Design review of the part built by this model. Coordinates are the model's own, in mm. A direction names the side the tool comes from. Coordinates: 2 decimals unless noted, no trailing zeros. Loops run counter-clockwise (first coordinate to the right, second up) from the corner with the lowest first, then second, coordinate; pieces in that order, holes last. Notation, with made-up numbers: (13.25, 79.5) -> (35.25, 79.5) arc R13 cw to (35.25, 89.5) -> close; hole circle Ø7 at (71.5, 0). An arc over 180 degrees is marked (long way). Use CSV: the item, a comma, the result in double quotes.
```python
from build123d import *

# Parameters (mm, degrees)
SKETCH1_W               = 95.25
SKETCH1_H               = 65.405
BOSS_EXTRUDE1_DEPTH     = 21.59
SKETCH2_W               = 90.17
SKETCH2_H               = 60.325
CUT_EXTRUDE1_DEPTH      = 21.59
CUT_EXTRUDE2_REACH      = 104.996
SKETCH3_W               = 7
SKETCH3_H               = 3
CUT_EXTRUDE3_DEPTH      = 84.738179763
CUT_EXTRUDE3_DEPTH_BACK = 84.738179763
SKETCH4_W               = 20.32
SKETCH4_H               = 3.81


with BuildPart() as part:
    # Sketch1 → Boss-Extrude1 (new body)
    with BuildSketch(Plane(origin=(0, 0, 0), x_dir=(1, 0, 0), z_dir=(0, 1, 0))):
        Rectangle(SKETCH1_W, SKETCH1_H)
    extrude(amount=BOSS_EXTRUDE1_DEPTH)

    # Sketch2 → Cut-Extrude1 (cut)
    with BuildSketch(Plane(origin=(0, 21.59, 0), x_dir=(1, 0, 0), z_dir=(0, 1, 0))):
        Rectangle(SKETCH2_W, SKETCH2_H)
    extrude(amount=-CUT_EXTRUDE1_DEPTH, mode=Mode.SUBTRACT)

    # Sketch3 → Cut-Extrude2 (cut, up to next)
    with BuildSketch(Plane.ZY.offset(47.625), mode=Mode.PRIVATE) as cut_extrude2_sk1:
        with Locations((0, 5.08)):
            Rectangle(SKETCH3_W, SKETCH3_H)
    cut_extrude2_tool1 = extrude(cut_extrude2_sk1.sketch, amount=-CUT_EXTRUDE2_REACH, mode=Mode.PRIVATE) & part.part
    add(cut_extrude2_tool1.solids().sort_by_distance((-47.625, 5.08, 0))[0], mode=Mode.SUBTRACT)

    # Sketch4 → Cut-Extrude3 (cut, two sides: drawn at the far end of the back side and taken through both)
    with BuildSketch(Plane(origin=(0, 0, -32.7025), x_dir=(-1, 0, 0), z_dir=(0, 0, -1)).offset(-CUT_EXTRUDE3_DEPTH_BACK)):
        with Locations((-31.115, 1.905)):
            Rectangle(SKETCH4_W, SKETCH4_H)
        with Locations((31.115, 1.905)):
            Rectangle(SKETCH4_W, SKETCH4_H)
    extrude(amount=CUT_EXTRUDE3_DEPTH + CUT_EXTRUDE3_DEPTH_BACK, mode=Mode.SUBTRACT)


solid = part.part
```
Item 1: Add section A-A (z = 5.5). Give the boundary of the cut face in (x, y) (3 decimals), then the cut area to 3 significant figures.
Checked values:
outline,"(-47.625, 0) -> (-45.085, 0) -> (-45.085, 21.59) -> (-47.625, 21.59) -> close; (45.085, 0) -> (47.625, 0) -> (47.625, 21.59) -> (45.085, 21.59) -> close"
area,"110 mm^2"
Item 2: Add section B-B (x = -25.5). Give the boundary of the cut face in (y, z).
Checked values:
outline,"(3.81, -32.7) -> (21.59, -32.7) -> (21.59, -30.16) -> (3.81, -30.16) -> close; (3.81, 30.16) -> (21.59, 30.16) -> (21.59, 32.7) -> (3.81, 32.7) -> close"
Item 3: Add section C-C (y = 12). Give the boundary of the cut face in (x, z) (1 decimal), then the cut area to 3 significant figures.
Checked values:
outline,"(-47.6, -32.7) -> (47.6, -32.7) -> (47.6, 32.7) -> (-47.6, 32.7) -> close; hole (-45.1, -30.2) -> (45.1, -30.2) -> (45.1, 30.2) -> (-45.1, 30.2) -> close"
area,"790 mm^2"
Item 4: Clearance check with a flat-ended pin moving along its axis: pin 1 (1.3 mm diameter, centred on x = -31, z = 31, fed in from -Y). State where the tip first meets the part, or that it passes through.
Checked values:
pin 1,"y = 3.81"
Item 5: To check wall thickness, follow line 1 along X through (y, z) = (5.25, 27) (3 decimals); line 2 along Z through (x, y) = (-17, 5). State the ranges of each line that lie inside material, in increasing order.
Checked values:
line 1,"-47.625 to -45.085, 45.085 to 47.625"
line 2,"-32.7 to -30.16, 30.16 to 32.7"
Item 6: Machinability: for faces 5 (the face through (-46, 5, 3.5)), 6 (the face through (-45.085, 11, 0)), 7 (the face through (-31, 3.81, 31)), 8 (the face through (47.625, 11, 0)), 9 (the face through (-47, 0, 0)), which of the approach directions +Z, -Z, +X, -X, +Y, -Y give a long, thin tool a straight path to every point of the face, cutting with its end or side? Answer none if there is none.
Checked values:
face 5,"-X"
face 6,"+Y, -Y"
face 7,"+Z, -Z, -Y"
face 8,"+Z, -Z, +X, +Y, -Y"
face 9,"+Z, -Z, +X, -X, -Y"
Item 7: Draft analysis for pull direction Z (two halves, no side actions). For faces 1 (the face through (-31, 3.81, -31)), 2 (the face through (45.085, 11, 0)), 3 (the face through (-1, 11, 32.702)), 4 (the face through (-1, 11, -32.702)), state which applies: pulls with the +Z half, pulls with the -Z half, needs draft (parallel to the pull), parting line crosses it, or undercut.
Checked values:
face 1,"needs draft"
face 2,"undercut"
face 3,"pulls with the +Z half"
face 4,"pulls with the -Z half"
